Source: CAD feature listing. Evaluate the final solid. Frame: model axes, mm. Face numbers are marked on the shaded views. A direction names the side the tool comes from. Give positions to 0.01 mm unless a question says otherwise; leave off trailing zeros. Loops run counter-clockwise (first coordinate to the right, second up) from the corner with the lowest first, then second, coordinate; pieces in that order, holes last.
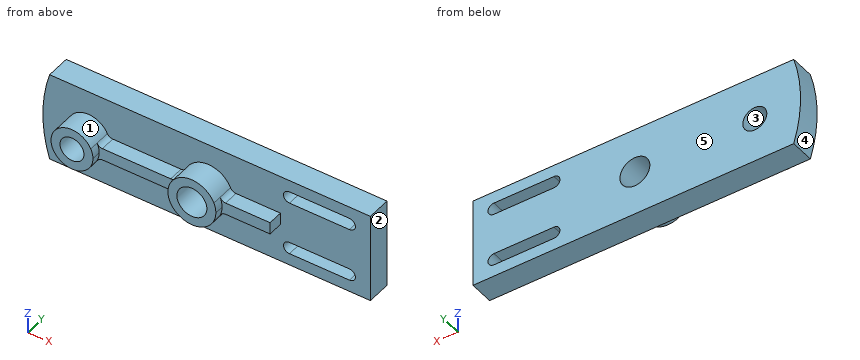
```python
from build123d import *

# Parameters (mm, degrees)
F1_DEPTH = 8
F2_DEPTH = 13
F0_R     = 4
F0_R_2   = 5
F3_DEPTH = 16


with BuildPart() as f1:
    # F0 (on Front) → F1 (new body)
    with BuildSketch(Plane.XZ):
        with BuildLine():
            Line((107, 0), (0, 0))
            ThreePointArc((0, 0), (-2.25577, -15), (0, -30))
            Line((0, -30), (107, -30))
            Line((107, -30), (107, 0))
        make_face()
        with BuildLine():
            ThreePointArc((80, -26), (78, -24), (80, -22))
            Line((80, -22), (100, -22))
            ThreePointArc((100, -22), (102, -24), (100, -26))
            Line((100, -26), (80, -26))
        make_face(mode=Mode.SUBTRACT)
        with BuildLine():
            ThreePointArc((19.270645, -18.111111), (6, -15), (19.270645, -11.888889))
            ThreePointArc((19.270645, -11.888889), (20.008165, -12.699673), (21.062258, -13))
            Line((21.062258, -13), (43.834849, -13))
            ThreePointArc((43.834849, -13), (44.930294, -12.67332), (45.667879, -11.8))
            ThreePointArc((45.667879, -11.8), (53, -7), (60.332121, -11.8))
            ThreePointArc((60.332121, -11.8), (61.069706, -12.67332), (62.165151, -13))
            Line((62.165151, -13), (77, -13))
            Line((77, -13), (77, -17))
            Line((77, -17), (62.165151, -17))
            ThreePointArc((62.165151, -17), (61.069706, -17.32668), (60.332121, -18.2))
            ThreePointArc((60.332121, -18.2), (53, -23), (45.667879, -18.2))
            ThreePointArc((45.667879, -18.2), (44.930294, -17.32668), (43.834849, -17))
            Line((43.834849, -17), (21.062258, -17))
            ThreePointArc((21.062258, -17), (20.008165, -17.300327), (19.270645, -18.111111))
        make_face(mode=Mode.SUBTRACT)
        with BuildLine():
            ThreePointArc((80, -8), (78, -6), (80, -4))
            Line((80, -4), (100, -4))
            ThreePointArc((100, -4), (102, -6), (100, -8))
            Line((100, -8), (80, -8))
        make_face(mode=Mode.SUBTRACT)
    extrude(amount=F1_DEPTH)

    # F0 (on Front) → F2 (join)
    with BuildSketch(Plane.XZ):
        with BuildLine():
            ThreePointArc((19.270645, -11.888889), (19.815222, -13.402269), (20, -15))
            ThreePointArc((20, -15), (19.815222, -16.597731), (19.270645, -18.111111))
            ThreePointArc((19.270645, -18.111111), (20.008165, -17.300327), (21.062258, -17))
            Line((21.062258, -17), (43.834849, -17))
            ThreePointArc((43.834849, -17), (44.930294, -17.32668), (45.667879, -18.2))
            ThreePointArc((45.667879, -18.2), (45, -15), (45.667879, -11.8))
            ThreePointArc((45.667879, -11.8), (44.930294, -12.67332), (43.834849, -13))
            Line((43.834849, -13), (21.062258, -13))
            ThreePointArc((21.062258, -13), (20.008165, -12.699673), (19.270645, -11.888889))
        make_face()
        with BuildLine():
            ThreePointArc((62.165151, -13), (61.069706, -12.67332), (60.332121, -11.8))
            ThreePointArc((60.332121, -11.8), (60.831251, -13.365523), (61, -15))
            ThreePointArc((61, -15), (60.831251, -16.634477), (60.332121, -18.2))
            ThreePointArc((60.332121, -18.2), (61.069706, -17.32668), (62.165151, -17))
            Line((62.165151, -17), (77, -17))
            Line((77, -17), (77, -13))
            Line((77, -13), (62.165151, -13))
        make_face()
    extrude(amount=F2_DEPTH)

    # F0 (on Front) → F3 (join)
    with BuildSketch(Plane.XZ):
        with BuildLine():
            ThreePointArc((19.270645, -18.111111), (19.815222, -16.597731), (20, -15))
            ThreePointArc((20, -15), (19.815222, -13.402269), (19.270645, -11.888889))
            ThreePointArc((19.270645, -11.888889), (6, -15), (19.270645, -18.111111))
        make_face()
        with Locations((13, -15)):
            Circle(F0_R, mode=Mode.SUBTRACT)
        with BuildLine():
            ThreePointArc((60.332121, -11.8), (53, -7), (45.667879, -11.8))
            ThreePointArc((45.667879, -11.8), (45, -15), (45.667879, -18.2))
            ThreePointArc((45.667879, -18.2), (53, -23), (60.332121, -18.2))
            ThreePointArc((60.332121, -18.2), (60.831251, -16.634477), (61, -15))
            ThreePointArc((61, -15), (60.831251, -13.365523), (60.332121, -11.8))
        make_face()
        with Locations((53, -15)):
            Circle(F0_R_2, mode=Mode.SUBTRACT)
    extrude(amount=F3_DEPTH)


solid = f1.part
```
(1) Section C-C, the plane z = -5.5. Return the cut outline in (x, y).
A:
outline: (-1.36, -8) - (78.06, -8) - (78.06, 0) - (-1.36, 0) - close; (101.94, -8) - (107, -8) - (107, 0) - (101.94, 0) - close
(2) Section A-A, the plane y = -9.25. Return the cut outline in (x, z), then the cut area to 3 significant figures.
A:
outline: (19.27, -18.11) arc R2 cw to (21.06, -17) - (43.83, -17) arc R2 cw to (45.67, -18.2) arc R8 ccw to (60.33, -18.2) arc R2 cw to (62.17, -17) - (77, -17) - (77, -13) - (62.17, -13) arc R2 cw to (60.33, -11.8) arc R8 ccw to (45.67, -11.8) arc R2 cw to (43.83, -13) - (21.06, -13) arc R2 cw to (19.27, -11.89) arc R7 ccw (long way) to start; hole circle Ø8 at (13, -15); hole circle Ø10 at (53, -15)
area: 393 mm2
(3) Mould query, pull axis Z, two halves, no side actions, for the marked faces 3, 4 and 5. Classes: pulls with the +Z half, pulls with the -Z half, needs draft (parallel to the pull), parting line crosses it, or undercut.
A:
face 3: undercut
face 4: parting line crosses it
face 5: needs draft
(4) Section D-D, the plane y = -4.75. Return the cut outline in (x, z).
A:
outline: (0, -30) - (107, -30) - (107, 0) - (0, 0) arc R51 ccw to start; hole circle Ø8 at (13, -15); hole circle Ø10 at (53, -15); hole (80, -26) - (100, -26) arc R2 ccw to (100, -22) - (80, -22) arc R2 ccw to start; hole (80, -8) - (100, -8) arc R2 ccw to (100, -4) - (80, -4) arc R2 ccw to start
(5) Section B-B, the plane x = 50. Return the cut outline in (y, z), then the cut area to 3 significant figures.
A:
outline: (-16, -22.42) - (-8, -22.42) - (-8, -30) - (0, -30) - (0, -19) - (-16, -19) - close; (-16, -11) - (0, -11) - (0, 0) - (-8, 0) - (-8, -7.58) - (-16, -7.58) - close
area: 231 mm2
(6) Reachability of the marked faces 1 and 2 from +Z, -Z, +X, -X, +Y, -Y: full face, straight path, thin tool, end or side. Return the list, or none.
A:
face 1: -Y
face 2: +Z, -Z, +X, +Y, -Y
(7) First-contact query: pin 1 (7 mm diameter, centred on x = 67, z = -15.5, fed in from -Y); pin 2 (2 mm diameter, centred on y = -5, z = -7.5, fed in from -X); pin 3 (2.5 mm diameter, centred on x = 32.5, y = -9.5, fed in from -Z); pin 4 (7 mm diameter, centred on x = 13, z = -15, fed in from -Y). Flat tips, straight axial feed; report the tip coordinate or a pass-through.
A:
pin 1: stops at y = -13
pin 2: stops at x = -1.84
pin 3: stops at z = -17
pin 4: passes through
(8) Ray query, line 1 along Z through (x, y) = (53, -4.5); line 2 along Z through (x, y) = (53, -10.5); line 3 along Y through (x, z) = (75, -25). Return the intervals inside material, ascending.
A:
line 1: z = -30 to -20, -10 to 0
line 2: z = -23 to -20, -10 to -7
line 3: y = -8 to 0
